Check sheet for the modelled part. Datum: model origin and axes. Units: mm. Round coordinates to 2 decimals unless told otherwise and drop trailing zeros. Loops run counter-clockwise (first coordinate to the right, second up) from the corner with the lowest first, then second, coordinate; pieces in that order, holes last. Notation, with made-up numbers: (-20, -38.75) -> (-6, -38.75) arc R25 cw to (-6, -19.75) -> close; hole circle Ø3 at (73.25, 61). An arc over 180 degrees is marked (long way). Return JSON: item names as keys, results as strings.
from build123d import *

# Parameters (mm, degrees)
F0_W     = 203.2
F0_H     = 165.1
F1_DEPTH = 3.175
F2_R     = 66.675
F3_DEPTH = 12.7


with BuildPart() as f1:
    # F0 (on Front) → F1 (new body)
    with BuildSketch(Plane.XZ):
        Rectangle(F0_W, F0_H)
    extrude(amount=F1_DEPTH)

    # F2 (on face) → F3 (cut, symmetric)
    with BuildSketch(Plane.XZ.offset(3.175)):
        Circle(F2_R)
    extrude(amount=F3_DEPTH, both=True, mode=Mode.SUBTRACT)


solid = f1.part
Q1. Section check A-A (z = 0). Record the boundary of the cut face in (x, y) (3 decimals).
Results list:
{"outline": "(-101.6, -3.175) -> (-66.675, -3.175) -> (-66.675, 0) -> (-101.6, 0) -> close; (66.675, -3.175) -> (101.6, -3.175) -> (101.6, 0) -> (66.675, 0) -> close"}
Q2. Section check B-B (x = 0). Record the boundary of the cut face in (y, z) (3 decimals).
Results list:
{"outline": "(-3.175, -82.55) -> (0, -82.55) -> (0, -66.675) -> (-3.175, -66.675) -> close; (-3.175, 66.675) -> (0, 66.675) -> (0, 82.55) -> (-3.175, 82.55) -> close"}
Q3. Material ranges on line 1 (Z direction, x = 0, y = -1.2) (3 decimals); line 2 (X direction, y = -2.6, z = 21); line 3 (X direction, y = -2.15, z = 10.5), recorded low to high.
Results list:
{"line 1": "-82.55 to -66.675, 66.675 to 82.55", "line 2": "-101.6 to -63.28, 63.28 to 101.6", "line 3": "-101.6 to -65.84, 65.84 to 101.6"}
Q4. Section check C-C (y = -2.05). Record the boundary of the cut face in (x, z) (3 decimals).
Results list:
{"outline": "(-101.6, -82.55) -> (101.6, -82.55) -> (101.6, 82.55) -> (-101.6, 82.55) -> close; hole circle Ø133.35 at (0, 0)"}
Q5. Draft check along Z on faces 1 (the cylindrical face through (63.596, -1.61, 20.027)), 2 (the flat face through (-69, -3.175, 1)). Enter one of: released by +Z, released by -Z, zero draft, split by the parting line, or undercut.
Results list:
{"face 1": "undercut", "face 2": "zero draft"}
